```python
from build123d import *

# Parameters (mm, degrees)
BOSS_EXTRUDE1_DEPTH     = 3.75
SKETCH2_W               = 17.7
SKETCH2_H               = 14.8
SKETCH2_H_2             = 17.5
SKETCH2_W_2             = 7.5
SKETCH2_H_3             = 22.5
SKETCH2_H_4             = 10
SKETCH2_W_3             = 26.4
SKETCH2_H_5             = 4.8
SKETCH2_W_4             = 11
SKETCH2_H_6             = 7.5
SKETCH2_W_5             = 10
SKETCH2_W_6             = 23.1
SKETCH2_H_7             = 7.843975032
SKETCH2_W_7             = 26.1
SKETCH2_W_8             = 5
SKETCH2_W_9             = 5.5
SKETCH2_H_8             = 5.25
BOSS_EXTRUDE2_DEPTH     = 12.5
SKETCH5_W               = 23.75
SKETCH5_H               = 2.5
CUT_EXTRUDE2_DEPTH      = 136.329459099
BOSS_EXTRUDE3_DEPTH     = 15
CHAMFER1_SIZE           = 3.75
CUT_EXTRUDE3_DEPTH      = 137.811814183
CUT_EXTRUDE3_DEPTH_BACK = 12.5
SKETCH7_W               = 0.25
SKETCH7_H               = 5.343975032
SKETCH7_W_2             = 0.1
SKETCH7_H_2             = 7.5
SKETCH7_H_3             = 15
SKETCH7_H_4             = 12.3
SKETCH7_H_5             = 4.8
CUT_EXTRUDE4_DEPTH      = 137.811814183
CUT_EXTRUDE4_DEPTH_BACK = 12.5
SKETCH9_W               = 17.45
SKETCH9_H               = 0.1
SKETCH9_H_2             = 0.25
SKETCH9_W_2             = 34.8
SKETCH9_W_3             = 55
SKETCH10_W              = 1.75
SKETCH10_H              = 50.6
SKETCH10_W_2            = 5
SKETCH10_H_2            = 14.906024968
BOSS_EXTRUDE5_DEPTH     = 12.5


with BuildPart() as part:
    # Sketch1 → Boss-Extrude1 (new body)
    with BuildSketch(Plane(origin=(0, 0, 0), x_dir=(1, 0, 0), z_dir=(0, 1, 0))):
        Polygon((40, 0), (95, 0), (95, 70), (71.25, 70), (71.25, 87.5), (47.5, 87.5), (47.5, 95), (23.75, 95), (23.75, 85), (0, 85), (0, 40), (40, 40), align=None)
    extrude(amount=BOSS_EXTRUDE1_DEPTH)

    # Sketch2 → Boss-Extrude2 (add)
    with BuildSketch(Plane(origin=(0, 3.75, 0), x_dir=(1, 0, 0), z_dir=(0, 1, 0))):
        with Locations((86.15, 62.6)):
            Rectangle(SKETCH2_W, SKETCH2_H)
        with Locations((62.4, 78.75)):
            Rectangle(SKETCH2_W, SKETCH2_H_2)
        with Locations((23.55, 51.25)):
            Rectangle(SKETCH2_W_2, SKETCH2_H_3)
        with Locations((38.65, 90)):
            Rectangle(SKETCH2_W, SKETCH2_H_4)
        with Locations((53.2, 2.4)):
            Rectangle(SKETCH2_W_3, SKETCH2_H_5)
        with Locations((45.5, 43.75)):
            Rectangle(SKETCH2_W_4, SKETCH2_H_6)
        with Locations((5, 51.25)):
            Rectangle(SKETCH2_W_5, SKETCH2_H_3)
        with Locations((11.55, 81.078012484)):
            Rectangle(SKETCH2_W_6, SKETCH2_H_7)
        with Locations((81.95, 2.4)):
            Rectangle(SKETCH2_W_7, SKETCH2_H_5)
        with Locations((32.3, 51.25)):
            Rectangle(SKETCH2_W_8, SKETCH2_H_3)
        with Locations((71.75, 30)):
            Rectangle(SKETCH2_W_9, SKETCH2_H_8)
    extrude(amount=BOSS_EXTRUDE2_DEPTH)

    # Sketch5 → Cut-Extrude2 (cut, through all)
    with BuildSketch(Plane.XZ):
        with Locations((11.875, -83.75)):
            Rectangle(SKETCH5_W, SKETCH5_H)
        with Locations((59.375, -86.25)):
            Rectangle(SKETCH5_W, SKETCH5_H)
        with Locations((35.625, -93.75)):
            Rectangle(SKETCH5_W, SKETCH5_H)
        with Locations((83.125, -68.75)):
            Rectangle(SKETCH5_W, SKETCH5_H)
    extrude(amount=-CUT_EXTRUDE2_DEPTH, mode=Mode.SUBTRACT)

    # Sketch6 → Boss-Extrude3 (add)
    with BuildSketch(Plane.XZ):
        with BuildLine():
            Line((59.15, -87.9), (57.5, -87.9))
            ThreePointArc((57.5, -87.9), (56.65, -88.75), (57.5, -89.6))
            Line((57.5, -89.6), (62.5, -89.6))
            ThreePointArc((62.5, -89.6), (63.35, -88.75), (62.5, -87.9))
            Line((62.5, -87.9), (60.85, -87.9))
            Line((60.85, -87.9), (60.85, -85))
            ThreePointArc((60.85, -85), (60, -84.15), (59.15, -85))
            Line((59.15, -85), (59.15, -87.9))
        make_face()
        with BuildLine():
            Line((37.1, -95.4), (38.75, -95.4))
            ThreePointArc((38.75, -95.4), (39.6, -96.25), (38.75, -97.1))
            Line((38.75, -97.1), (33.75, -97.1))
            ThreePointArc((33.75, -97.1), (32.9, -96.25), (33.75, -95.4))
            Line((33.75, -95.4), (35.4, -95.4))
            Line((35.4, -95.4), (35.4, -92.5))
            ThreePointArc((35.4, -92.5), (36.25, -91.65), (37.1, -92.5))
            Line((37.1, -92.5), (37.1, -95.4))
        make_face()
        with BuildLine():
            Line((13.35, -85.4), (15, -85.4))
            ThreePointArc((15, -85.4), (15.85, -86.25), (15, -87.1))
            Line((15, -87.1), (10, -87.1))
            ThreePointArc((10, -87.1), (9.15, -86.25), (10, -85.4))
            Line((10, -85.4), (11.65, -85.4))
            Line((11.65, -85.4), (11.65, -82.5))
            ThreePointArc((11.65, -82.5), (12.5, -81.65), (13.35, -82.5))
            Line((13.35, -82.5), (13.35, -85.4))
        make_face()
        with BuildLine():
            Line((81.25, -70.4), (82.9, -70.4))
            Line((82.9, -70.4), (82.9, -67.5))
            ThreePointArc((82.9, -67.5), (83.75, -66.65), (84.6, -67.5))
            Line((84.6, -67.5), (84.6, -70.4))
            Line((84.6, -70.4), (86.25, -70.4))
            ThreePointArc((86.25, -70.4), (87.1, -71.25), (86.25, -72.1))
            Line((86.25, -72.1), (81.25, -72.1))
            ThreePointArc((81.25, -72.1), (80.4, -71.25), (81.25, -70.4))
        make_face()
    extrude(amount=-BOSS_EXTRUDE3_DEPTH)

    # Chamfer1
    # the kernel refuses this chamfer: 3.75 mm, written as the material it takes off along each edge
    with BuildSketch(Plane(origin=(47.856188795, 15, -89.6), x_dir=(0, 0.027495876610586334, 0.9996219169112968), z_dir=(1, 0, 0))) as chamfer1_piece_1:
        Polygon((CHAMFER1_SIZE * 0.999621916911, CHAMFER1_SIZE * 0.0274958766106), (-CHAMFER1_SIZE * 0.0274958766106, CHAMFER1_SIZE * 0.999621916911), (0, 0), align=None)
    extrude(amount=24.28762241, mode=Mode.SUBTRACT)
    with BuildSketch(Plane(origin=(48.393811205, 15, -97.1), x_dir=(0, 0.027495876610586334, 0.9996219169112968), z_dir=(-1, 0, 0)), Plane(origin=(95.893811205, 15, -72.1), x_dir=(0, 0.027495876610586334, 0.9996219169112968), z_dir=(-1, 0, 0)), Plane(origin=(24.643811205, 15, -87.1), x_dir=(0, 0.027495876610586334, 0.9996219169112968), z_dir=(-1, 0, 0))) as chamfer1_piece_2:
        Polygon((CHAMFER1_SIZE * 0.999621916911, -CHAMFER1_SIZE * 0.0274958766106), (-CHAMFER1_SIZE * 0.0274958766106, -CHAMFER1_SIZE * 0.999621916911), (0, 0), align=None)
    extrude(amount=24.28762241, mode=Mode.SUBTRACT)

    # Sketch7 → Cut-Extrude3 (cut, two sides: drawn at the far end of the back side and taken through both)
    with BuildSketch(Plane(origin=(0, 16.25, 0), x_dir=(1, 0, 0), z_dir=(0, 1, 0)).offset(-CUT_EXTRUDE3_DEPTH_BACK)):
        with Locations((22.975, 79.828012484)):
            Rectangle(SKETCH7_W, SKETCH7_H)
        with Locations((29.85, 88.75)):
            Rectangle(SKETCH7_W_2, SKETCH7_H_2)
        Polygon((29.8, 62.5), (29.9, 62.5), (29.9, 55), (34.8, 55), (34.8, 40), (0, 40), (0, 55), (29.8, 55), align=None)
        with Locations((53.675, 77.5)):
            Rectangle(SKETCH7_W, SKETCH7_H_3)
        with Locations((40.125, 43.75)):
            Rectangle(SKETCH7_W, SKETCH7_H_2)
        with Locations((77.425, 61.35)):
            Rectangle(SKETCH7_W, SKETCH7_H_4)
        with Locations((69.025, 2.4)):
            Rectangle(SKETCH7_W, SKETCH7_H_5)
    extrude(amount=CUT_EXTRUDE3_DEPTH + CUT_EXTRUDE3_DEPTH_BACK, mode=Mode.SUBTRACT)

    # Sketch9 → Cut-Extrude4 (cut, two sides: drawn at the far end of the back side and taken through both)
    with BuildSketch(Plane(origin=(0, 16.25, 0), x_dir=(1, 0, 0), z_dir=(0, 1, 0)).offset(-CUT_EXTRUDE4_DEPTH_BACK)):
        with Locations((86.275, 55.25)):
            Rectangle(SKETCH9_W, SKETCH9_H)
        with Locations((62.525, 70.125)):
            Rectangle(SKETCH9_W, SKETCH9_H_2)
        with Locations((17.4, 62.375)):
            Rectangle(SKETCH9_W_2, SKETCH9_H_2)
        with Locations((67.5, 4.75)):
            Rectangle(SKETCH9_W_3, SKETCH9_H)
    extrude(amount=CUT_EXTRUDE4_DEPTH + CUT_EXTRUDE4_DEPTH_BACK, mode=Mode.SUBTRACT)

    # Sketch10 → Boss-Extrude5 (add)
    with BuildSketch(Plane(origin=(0, 3.75, 0), x_dir=(1, 0, 0), z_dir=(0, 1, 0))):
        with Locations((94.125, 30)):
            Rectangle(SKETCH10_W, SKETCH10_H)
        with Locations((2.5, 69.703012484)):
            Rectangle(SKETCH10_W_2, SKETCH10_H_2)
    extrude(amount=BOSS_EXTRUDE5_DEPTH)


solid = part.part
```
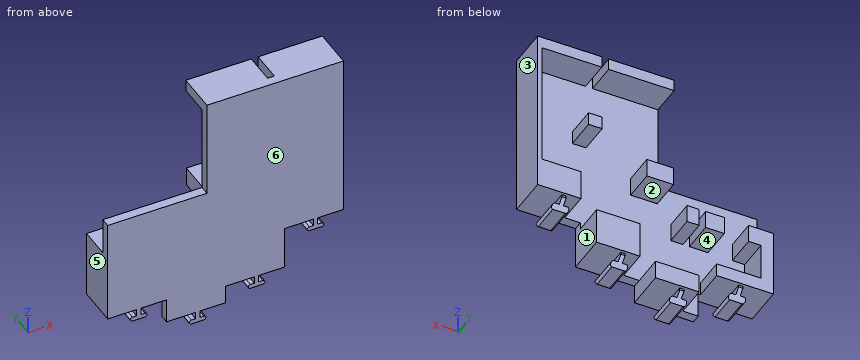
Geometry: final body of the model. Coordinates: model frame, mm. Face numbers are marked on the shaded views. A direction names the side the tool comes from. Coordinates: 2 decimals unless noted, no trailing zeros. Loops run counter-clockwise (first coordinate to the right, second up) from the corner with the lowest first, then second, coordinate; pieces in that order, holes last. Notation, with made-up numbers: (51.25, 10) -> (62.25, 10) arc R26 ccw to (62.25, 31) -> close; hole circle Ø6 at (89.25, -0.75). An arc over 180 degrees is marked (long way). Use a Markdown table: item, result. Add a question column.
(1) Section query C-C, the plane y = 5.25. State how many separate pieces and enclosed holes the cut face has, plus the area to 3 significant figures.
(2) Access query for the marked faces 1, 2 and 3. Directions: +Z, -Z, +X, -X, +Y, -Y. A direction counts if a zero-diameter tool reaches every point of the face in a straight line with its end or side. Return the directions, or none.
(3) Section query D-D, the plane z = -65.5. Return loops of the section in (x, y).
(4) Line query: line 1 along Z through (x, y) = (89, 8.5); line 2 along X through (y, z) = (12.25, -65.5); line 3 along Z through (x, y) = (9, 10). Output: solid intervals per line, ascending.
(5) Section query B-B, the plane x = 17. Return loops of the section in (y, z).
(6) Pin query (flat end, axial travel): pin 1 Ø8 at (x, y) = (6.5, 12.5) entering from +Z; pin 2 Ø5 at (x, y) = (57.5, 8.5) entering from -Z; pin 3 Ø1.6 at (x, y) = (70.5, 10.5) entering from -Z. Return the tip coordinate at first contact, or that it passes through.
(7) Mould query, pull axis X, two halves, no side actions, for the marked faces 4, 5 and 6. Classes: pulls with the +X half, pulls with the -X half, needs draft (parallel to the pull), parting line crosses it, or undercut.
(8) Section query A-A, the plane z = -45. Return loops of the section in (x, y), plus the area to 4 significant figures.
Answer:
| question | item | result |
|---|---|---|
| 1 | separate pieces | 9 |
| 1 | enclosed holes | 0 |
| 1 | area | 1,470 mm^2 |
| 2 | face 1 | -Z, +Y, -Y |
| 2 | face 2 | -X, +Y |
| 2 | face 3 | +Z, -Z, +X, +Y, -Y |
| 3 | outline | (0, 0) -> (95, 0) -> (95, 16.25) -> (77.55, 16.25) -> (77.55, 3.75) -> (5, 3.75) -> (5, 16.25) -> (0, 16.25) -> close |
| 4 | line 1 | z = -67.5 to -55.3, -4.7 to 0 |
| 4 | line 2 | x = 0 to 5, 77.55 to 95 |
| 4 | line 3 | z = -82.5 to -77.16, -62.25 to -55 |
| 5 | outline | (0, -82.5) -> (16.25, -82.5) -> (16.25, -77.16) -> (3.75, -77.16) -> (3.75, -40) -> (0, -40) -> close |
| 6 | pin 1 | stops at z = -55 |
| 6 | pin 2 | stops at z = -89.6 |
| 6 | pin 3 | stops at z = -85 |
| 7 | face 4 | undercut |
| 7 | face 5 | pulls with the -X half |
| 7 | face 6 | needs draft |
| 8 | outline | (0, 0) -> (95, 0) -> (95, 16.25) -> (93.25, 16.25) -> (93.25, 3.75) -> (51, 3.75) -> (51, 16.25) -> (40.25, 16.25) -> (40.25, 3.75) -> (0, 3.75) -> close |
| 8 | area | 512.5 mm^2 |
